```python
from build123d import *

# Parameters (mm, degrees)
SKETCH1_W           = 240
SKETCH1_H           = 112
BOSS_EXTRUDE1_DEPTH = 70
SKETCH2_W           = 180
SKETCH2_H           = 52
CUT_EXTRUDE1_DEPTH  = 10
CUT_EXTRUDE1_TAPER  = 20
FILLET1_R           = 5


with BuildPart() as part:
    # Sketch1 → Boss-Extrude1 (new body)
    with BuildSketch(Plane(origin=(0, 0, 0), x_dir=(1, 0, 0), z_dir=(0, 1, 0))):
        Rectangle(SKETCH1_W, SKETCH1_H)
    extrude(amount=BOSS_EXTRUDE1_DEPTH)

    # Sketch2 → Cut-Extrude1 (cut)
    with BuildSketch(Plane(origin=(0, 70, 0), x_dir=(1, 0, 0), z_dir=(0, 1, 0))):
        Rectangle(SKETCH2_W, SKETCH2_H)
    cut_extrude1 = extrude(amount=-CUT_EXTRUDE1_DEPTH, taper=CUT_EXTRUDE1_TAPER, mode=Mode.SUBTRACT)

    # Mirror1: Cut-Extrude1 across plane
    add(cut_extrude1.mirror(Plane.ZX.offset(35)), mode=Mode.SUBTRACT)

    # Fillet1
    fillet1_edges = [part.edges().sort_by_distance(p)[0] for p in [
        (86.360297657, 60, 0),
        (0, 60, 22.360297657),
        (-86.360297657, 60, 0),
        (0, 60, -22.360297657),
        (90, 70, 0),
        (0, 70, -26),
        (-90, 70, 0),
        (0, 70, 26),
        (90, 0, 0),
        (0, 0, -26),
        (-90, 0, 0),
        (0, 0, 26),
        (86.360297657, 10, 0),
        (0, 10, -22.360297657),
        (-86.360297657, 10, 0),
        (0, 10, 22.360297657),
    ]]
    fillet(fillet1_edges, radius=FILLET1_R)


solid = part.part
```
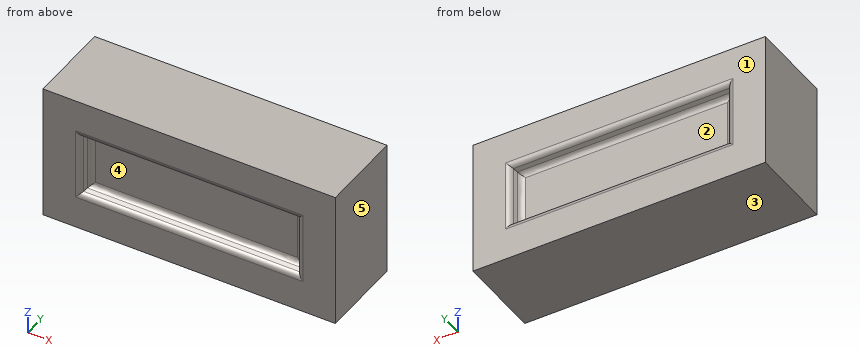
Can you work these out from the model? Positions are in its coordinate system, mm. Face numbers are marked on the shaded views. A direction names the side the tool comes from. Round coordinates to 2 decimals unless told otherwise and drop trailing zeros. Return JSON: item names as keys, results as strings. Group by question number.
1. Which directions (+Z, -Z, +X, -X, +Y, -Y) give clear straight access to the entire face, cutting with the end or side of a thin tool? Please do the marked faces 1 and 2.
2. I need wall thicknesses on line 1 (Y direction, x = 18.5, z = 11.5); line 2 (X direction, y = 64.5, z = -10); line 3 (Z direction, x = 43, y = 8.5). Which ranges of each line are inside material? Lowest first, please. Write a range as [from, to].
3. We'd pull the mould along Z, two halves only. Please class the marked faces 3, 4 and 5: released by +Z, released by -Z, zero draft, split by the parting line, or undercut.
4. Will these pins go through, and if not, where does the flat tip stop? pin 1 (8 mm diameter, centred on x = 33.5, z = 2.5, fed in from +Y); pin 2 (11.5 mm diameter, centred on x = -39.5, z = 4.5, fed in from -Y); pin 3 (4 mm diameter, centred on x = 69.5, z = -21, fed in from -Y).
Output values:
{
 "1": {"face 1": "+Z, -Z, +X, -X, +Y", "face 2": "+Y"},
 "2": {"line 1": "[10, 60]", "line 2": "[-120, -88], [88, 120]", "line 3": "[-56, -22.43], [22.43, 56]"},
 "3": {"face 3": "released by -Z", "face 4": "undercut", "face 5": "zero draft"},
 "4": {"pin 1": "y = 60", "pin 2": "y = 10", "pin 3": "y = 7.8"}
}
